For this review, use the dimensioned drawing (mm, ordinates from the lowest corner) and the shaded views. Coordinates: 2 decimals unless noted, no trailing zeros. Loops run counter-clockwise (first coordinate to the right, second up) from the corner with the lowest first, then second, coordinate; pieces in that order, holes last. Notation, with made-up numbers: M 7.25,2 L 34.25,2 A5 cw 34.25,7 Z; hole C 84,55 d7. An arc over 180 degrees is marked long. One line per item, written item: value.
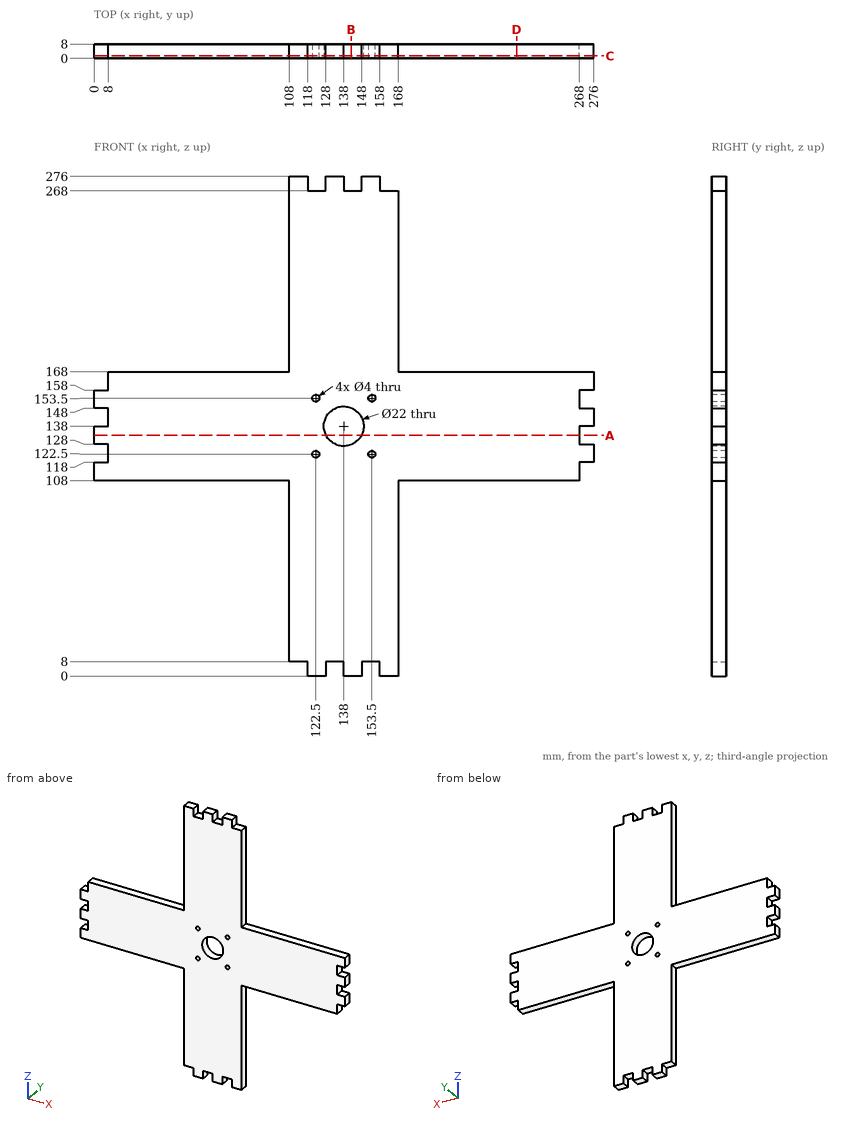
(1) Add section B-B on x = 142. State the section outline as (y, z) points.
Checks:
outline: M 0,0 L 8,0 L 8,127.75 L 0,127.75 Z; M 0,148.25 L 8,148.25 L 8,268 L 0,268 Z
(2) To check wall thickness, follow L1, parallel to X at y = 5.25, z = 153.5; L2, parallel to Z at x = 153.5, y = 6.75. State the ranges of each line that lie inside material, in increasing order. Write a range as [from, to].
Checks:
L1: [0, 120.5], [124.5, 151.5], [155.5, 268]
L2: [8, 120.5], [124.5, 151.5], [155.5, 276]
(3) Add section C-C on y = 1.5. State how many separate pieces and enclosed holes the cut face has, then the cut area to 3 significant figures.
Checks:
separate pieces: 1
enclosed holes: 5
area: 28,100 mm^2
(4) Add section A-A on z = 133. State the section outline as (x, y) points.
Checks:
outline: M 0,0 L 128.2,0 L 128.2,8 L 0,8 Z; M 147.8,0 L 268,0 L 268,8 L 147.8,8 Z
(5) Add section D-D on x = 233.5. State the section outline as (y, z) points, then the cut area to 3 significant figures.
Checks:
outline: M 0,108 L 8,108 L 8,168 L 0,168 Z
area: 480 mm^2
(6) Insertion check: pin 1 Ø4 at (y, z) = (6, 124.5) entering from -X; pin 2 Ø4 at (x, y) = (272.5, 4.5) entering from -Z; pin 3 Ø2.5 at (x, y) = (56, 4.5) entering from +Z. Each pin has a flat end and moves straight along its axis. Give the tip position at first contact, or say it passes through.
Checks:
pin 1: x = 8
pin 2: z = 118
pin 3: z = 168
